from build123d import *

# Parameters (mm, degrees)
CUT_EXTRUDE_1_DEPTH = 3
CHAMFER_1_SIZE      = 0.25


with BuildPart() as part:
    # Эскиз1 → Повернуть1 (revolve)
    with BuildSketch(Plane.XY):
        with BuildLine():
            Line((-4.982457352, 2.5), (-5.3, 3.05))
            Line((-5.3, 3.05), (-5.3, 5))
            Line((-5.3, 5), (0, 5))
            Line((0, 5), (0, 3.4))
            ThreePointArc((0, 3.4), (0.046179295, 3.255234258), (0.167656961, 3.163949955))
            Line((0.167656961, 3.163949955), (0.597656961, 3.013949955))
            ThreePointArc((0.597656961, 3.013949955), (0.638241835, 3.003512159), (0.68, 3))
            Line((0.68, 3), (25, 3))
            Line((25, 3), (25, 0))
            Line((25, 0), (-0.856624327, 0))
            Line((-0.856624327, 0), (-2.3, 2.5))
            Line((-2.3, 2.5), (-4.982457352, 2.5))
        make_face()
    revolve(axis=Axis((-1000, 0, 0), (1, 0, 0)))

    # Эскиз2 → Вырез-Вытянуть1 (cut)
    with BuildSketch(Plane.ZY.offset(5.3)):
        with BuildLine():
            Line((-0.038113557, 2.864746473), (-2.461886443, 1.465380546))
            ThreePointArc((-2.461886443, 1.465380546), (-2.481162782, 1.4325), (-2.5, 1.399365928))
            Line((-2.5, 1.399365928), (-2.5, -1.399365928))
            ThreePointArc((-2.5, -1.399365928), (-2.481162782, -1.4325), (-2.461886443, -1.465380546))
            Line((-2.461886443, -1.465380546), (-0.038113557, -2.864746473))
            ThreePointArc((-0.038113557, -2.864746473), (0, -2.865), (0.038113557, -2.864746473))
            Line((0.038113557, -2.864746473), (2.461886443, -1.465380546))
            ThreePointArc((2.461886443, -1.465380546), (2.481162782, -1.4325), (2.5, -1.399365928))
            Line((2.5, -1.399365928), (2.5, 1.399365928))
            ThreePointArc((2.5, 1.399365928), (2.481162782, 1.4325), (2.461886443, 1.465380546))
            Line((2.461886443, 1.465380546), (0.038113557, 2.864746473))
            ThreePointArc((0.038113557, 2.864746473), (0, 2.865), (-0.038113557, 2.864746473))
        make_face()
    extrude(amount=-CUT_EXTRUDE_1_DEPTH, mode=Mode.SUBTRACT)

    # Фаска1
    chamfer_1_edges = [part.edges().sort_by_distance(p)[0] for p in [
        (-5.3, -5, 0),
        (0, -5, 0),
        (25, -3, 0),
    ]]
    chamfer(chamfer_1_edges, length=CHAMFER_1_SIZE)


solid = part.part
The model under review builds one solid part; all positions refer to its coordinate system, in mm. A direction names the side the tool comes from. Give positions to 0.01 mm unless a question says otherwise; leave off trailing zeros. Write each loop counter-clockwise with the first axis right and the second up, starting at its lowest first coordinate (ties: lowest second). Pieces come first, ordered by that corner, then holes. Notation, with made-up numbers: M 39,27 L 85,27 A33 cw 85,60 Z; hole C 54.5,-17.5 d10. An arc over 180 degrees is marked long. One line per question, with ' | ' between items. Start each with the question number.
Item 1: Draft analysis for pull direction Z (two halves, no side actions). For faces 4 (the flat face through (-2.3, 1.328, -2.295)), 5 (the flat face through (25, 0, 0)), 6 (the cylindrical face through (13, -3, 0)), state which applies: released by +Z, released by -Z, zero draft, split by the parting line, or undercut.
Item 2: We need section A-A on x = 21. Write out the cut boundary in (y, z).
Item 3: For pin 1 (3 mm diameter, centred on x = 12.5, z = -4, fed in from +Y); pin 2 (1.4 mm diameter, centred on y = 1, z = 2, fed in from -X); pin 3 (0.6 mm diameter, centred on y = -0.5, z = 1.5, fed in from -X), all flat-tipped, find the tip position at first contact; note any pin that passes through.
Item 4: For faces 1 (the flat face through (-4, 0, -2.5)), 2 (the cylindrical face through (-2.62, -1.08, -4.88)), 3 (the flat face through (0, 2, -3)), list the 3-axis set-ups (+Z, -Z, +X, -X, +Y, -Y) from which the entire face can be reached by the end or side of a thin tool; tool diameter is ignored.
Item 5: Wall thickness on line 1 (X direction, y = 1.75, z = 4.25); line 2 (Z direction, x = -1.5, y = -0.25); line 3 (X direction, y = 2.25, z = -0.25): over which ranges is each line inside the solid? List them lowest first. Write a range as from..to.
Results found:
1) face 4: undercut | face 5: zero draft | face 6: split by the parting line
2) outline: C 0,0 d6
3) pin 1: stops at y = 1.66 | pin 2: stops at x = -5.23 | pin 3: stops at x = -1.94
4) face 1: -X | face 2: +X, -X | face 3: +X
5) line 1: x = -5.3..0 | line 2: z = -4.99..-1.09, 1.09..4.99 | line 3: x = -2.16..25
